Could you check a few things on this model? Use its own coordinates, in mm. Face numbers are marked on the shaded views. A direction names the side the tool comes from. Coordinates: 2 decimals unless noted, no trailing zeros. Order: outer loops, then holes, each group sorted by start corner. A loop starts at its lowest first (then second) coordinate and runs counter-clockwise, first axis right, second up. Notation, with made-up numbers: (28, 21.5) - (40, 21.5) arc R23 ccw to (40, 30.5) - close; hole circle Ø1 at (54.5, 5.25). An arc over 180 degrees is marked (long way). Answer as CSV lines item,"result". Start each with the question number.
1. Thinking about a two-plate mould opening in X: for the marked faces 1, 2, 3 and 4, which applies, released by +X, released by -X, zero draft, split by the parting line, or undercut?
2. I want a section at D-D, the plane y = -6.5. List the corners of the cut face in (x, z) for me.
3. I want a section at C-C, the plane y = -1. List the corners of the cut face in (x, z) for me, and give its area (3 significant figures).
4. For pin 1 (6 mm diameter, centred on y = 4.5, z = 10, fed in from -X); pin 2 (3.5 mm diameter, centred on x = 21.75, z = 25, fed in from +Y); pin 3 (7 mm diameter, centred on x = -21.75, z = 5, fed in from +Y); pin 4 (2 mm diameter, centred on x = -21, z = 10.5, fed in from +Y), each with a flat end and sliding along its axis, tell me the tip position at first contact or that it passes through.
5. For the marked faces 5, 6 and 7, which set-ups out of +Z, -Z, +X, -X, +Y, -Y let a thin tool reach every point of the face, with its end or its side?
6. I want a section at B-B, the plane x = 21.75. List the corners of the cut face in (y, z) for me.
7. I want a section at A-A, the plane z = 5. List the corners of the cut face in (x, y) for me, and give its area (3 significant figures).
8. I need wall thicknesses on probe 1 along X at (y, z) = (-8.2, 5); probe 2 along Z at (x, y) = (21.75, -7.65); probe 3 along X at (y, z) = (-2, 11). Which ranges of each line are inside material? Lowest first, please.
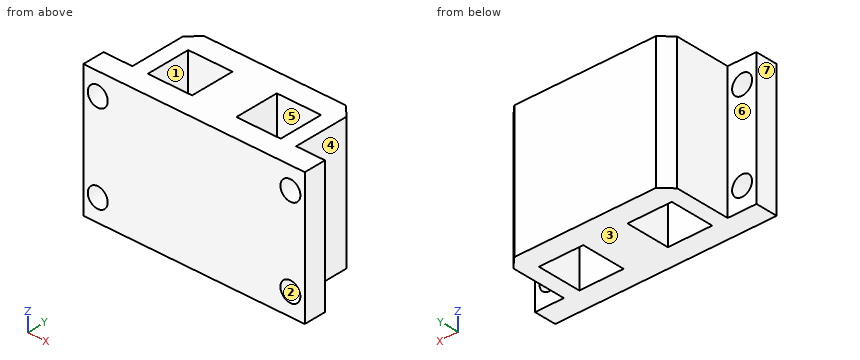
from build123d import *

# Parameters (mm, degrees)
SKETCH2_W           = 10
SKETCH2_H           = 10
BOSS_EXTRUDE1_DEPTH = 30
CHAMFER1_SIZE       = 2.5
SKETCH3_R           = 2.25
CUT_EXTRUDE1_DEPTH  = 6


with BuildPart() as part:
    # Sketch2 → Boss-Extrude1 (new body)
    with BuildSketch(Plane.XY):
        Polygon((-25, -10), (25, -10), (25, -5), (18.5, -5), (18.5, 10), (-18.5, 10), (-18.5, -5), (-25, -5), align=None)
        with Locations((-10, 0)):
            Rectangle(SKETCH2_W, SKETCH2_H, mode=Mode.SUBTRACT)
        with Locations((10, 0)):
            Rectangle(SKETCH2_W, SKETCH2_H, mode=Mode.SUBTRACT)
    extrude(amount=BOSS_EXTRUDE1_DEPTH)

    # Chamfer1
    chamfer1_edges = [part.edges().sort_by_distance(p)[0] for p in [
        (-18.5, 10, 15),
        (18.5, 10, 15),
    ]]
    chamfer(chamfer1_edges, length=CHAMFER1_SIZE)

    # Sketch3 → Cut-Extrude1 (cut, through all)
    with BuildSketch(Plane(origin=(0, -5, 0), x_dir=(1, 0, 0), z_dir=(0, 1, 0))):
        with Locations((-21.75, -5)):
            Circle(SKETCH3_R)
        with Locations((-21.75, -25)):
            Circle(SKETCH3_R)
        with Locations((21.75, -25)):
            Circle(SKETCH3_R)
        with Locations((21.75, -5)):
            Circle(SKETCH3_R)
    extrude(amount=-CUT_EXTRUDE1_DEPTH, mode=Mode.SUBTRACT)


solid = part.part
Solved:
1,face 1,"undercut"
1,face 2,"undercut"
1,face 3,"zero draft"
1,face 4,"released by +X"
2,outline,"(-25, 0) - (25, 0) - (25, 30) - (-25, 30) - close; hole circle Ø4.5 at (-21.75, 5); hole circle Ø4.5 at (-21.75, 25); hole circle Ø4.5 at (21.75, 5); hole circle Ø4.5 at (21.75, 25)"
3,outline,"(-18.5, 0) - (-15, 0) - (-15, 30) - (-18.5, 30) - close; (-5, 0) - (5, 0) - (5, 30) - (-5, 30) - close; (15, 0) - (18.5, 0) - (18.5, 30) - (15, 30) - close"
3,area,"510 mm2"
4,pin 1,"stops at x = -18.5"
4,pin 2,"passes through"
4,pin 3,"stops at y = 7.75"
4,pin 4,"stops at y = -5"
5,face 5,"+Z, -Z"
5,face 6,"+Z, -Z, -X, +Y"
5,face 7,"+Z, -Z, -X, +Y, -Y"
6,outline,"(-10, 0) - (-5, 0) - (-5, 2.75) - (-10, 2.75) - close; (-10, 7.25) - (-5, 7.25) - (-5, 22.75) - (-10, 22.75) - close; (-10, 27.25) - (-5, 27.25) - (-5, 30) - (-10, 30) - close"
7,outline,"(-25, -10) - (-24, -10) - (-24, -5) - (-25, -5) - close; (-19.5, -10) - (19.5, -10) - (19.5, -5) - (18.5, -5) - (18.5, 7.5) - (16, 10) - (-16, 10) - (-18.5, 7.5) - (-18.5, -5) - (-19.5, -5) - close; (24, -10) - (25, -10) - (25, -5) - (24, -5) - close; hole (-15, -5) - (-5, -5) - (-5, 5) - (-15, 5) - close; hole (5, -5) - (15, -5) - (15, 5) - (5, 5) - close"
7,area,"554 mm2"
8,probe 1,"x = -25 to -24, -19.5 to 19.5, 24 to 25"
8,probe 2,"z = 0 to 2.75, 7.25 to 22.75, 27.25 to 30"
8,probe 3,"x = -18.5 to -15, -5 to 5, 15 to 18.5"
